from build123d import *

# Parameters (mm, degrees)
F0_W     = 152.4
F0_H     = 152.4
F0_R     = 3.175
F0_R_2   = 6.35
F1_DEPTH = 3.175
F2_R     = 5.08
F3_R     = 19.044803008
F3_R_2   = 6.35
F4_DEPTH = 0.7055555556


# Not quite as in the source:
# - a length typed as a fraction of an inch, garbled in the dataset ("3 / 203.2 mm" for 3/8 in), is restored


with BuildPart() as f1:
    # F0 (on Top) → F1 (new body)
    with BuildSketch(Plane.XY):
        with Locations((-1.8146978691, -1.1040684107)):
            Rectangle(F0_W, F0_H)
        with Locations((-67.6762834191, -67.5093614922)):
            Circle(F0_R, mode=Mode.SUBTRACT)
        with Locations((65.6737165809, -67.5093614922)):
            Circle(F0_R, mode=Mode.SUBTRACT)
        with Locations((-67.6762834191, 65.8406385078)):
            Circle(F0_R, mode=Mode.SUBTRACT)
        Circle(F0_R_2, mode=Mode.SUBTRACT)
        with Locations((65.6737165809, 65.8406385078)):
            Circle(F0_R, mode=Mode.SUBTRACT)
    extrude(amount=F1_DEPTH)

    # F2
    f2_edges = [f1.edges().sort_by_distance(p)[0] for p in [
        (74.385302, 75.095932, 1.5875),
        (-78.014698, 75.095932, 1.5875),
        (74.385302, -77.304068, 1.5875),
        (-78.014698, -77.304068, 1.5875),
    ]]
    fillet(f2_edges, radius=F2_R)

    # F3 (on face) → F4 (cut)
    with BuildSketch(Plane.XY.offset(3.175)):
        Circle(F3_R)
        Circle(F3_R_2, mode=Mode.SUBTRACT)
    extrude(amount=-F4_DEPTH, mode=Mode.SUBTRACT)


solid = f1.part
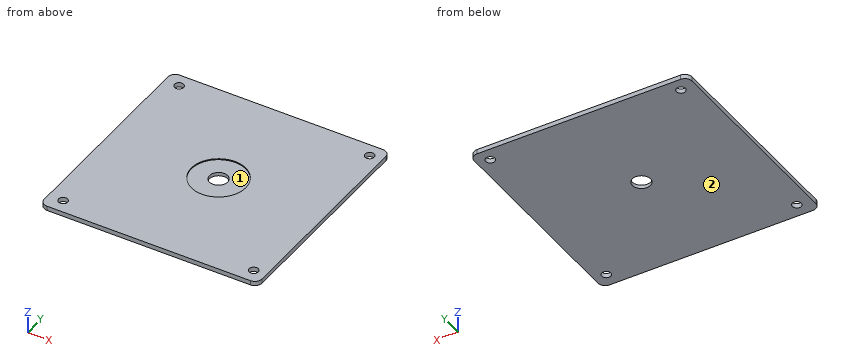
Can you work these out from the model? Positions are in its coordinate system, mm. Face numbers are marked on the shaded views. Round coordinates to 2 decimals unless told otherwise and drop trailing zeros. Write each loop counter-clockwise with the first axis right and the second up, starting at its lowest first coordinate (ties: lowest second). Pieces come first, ordered by that corner, then holes. Notation, with made-up numbers: M 42.25,-31 L 86.25,-31 A17 ccw 86.25,-10 Z; hole C 55,11.5 d6. An arc over 180 degrees is marked long. Use a Markdown table: item, result.
Item 1: For pin 1 Ø1.5 at (x, y) = (8, 11.5) entering from +Z, with a flat end and sliding along its axis, tell me the tip position at first contact or that it passes through.
Found:
| item | result |
|---|---|
| pin 1 | stops at z = 2.47 |
Item 2: If I drill on line 1 along Y through (x, z) = (-65.5, 2.65); line 2 along Y through (x, z) = (0, 1.55); line 3 along X through (y, z) = (8, 2.85), over which ranges is the centre line in solid material (lowest first)? Write a range as [from, to].
Found:
| item | result |
|---|---|
| line 1 | y = [-77.3, -69.82], [-65.2, 63.53], [68.15, 75.1] |
| line 2 | y = [-77.3, -6.35], [6.35, 75.1] |
| line 3 | x = [-78.01, -17.28], [17.28, 74.39] |
Item 3: I want a section at A-A (y = 0). List the corners of the cut face in (x, z) for me (3 decimals), and give its area (3 significant figures).
Found:
| item | result |
|---|---|
| outline | M -78.015,0 L -6.35,0 L -6.35,2.469 L -19.045,2.469 L -19.045,3.175 L -78.015,3.175 Z; M 6.35,0 L 74.385,0 L 74.385,3.175 L 19.045,3.175 L 19.045,2.469 L 6.35,2.469 Z |
| area | 426 mm2 |
Item 4: We'd pull the mould along X, two halves only. Please class the marked faces 1 and 2: released by +X, released by -X, zero draft, split by the parting line, or undercut.
Found:
| item | result |
|---|---|
| face 1 | undercut |
| face 2 | zero draft |
Item 5: I want a section at B-B (x = 0). List the corners of the cut face in (y, z) for me (3 decimals), and give its area (3 significant figures).
Found:
| item | result |
|---|---|
| outline | M -77.304,0 L -6.35,0 L -6.35,2.469 L -19.045,2.469 L -19.045,3.175 L -77.304,3.175 Z; M 6.35,0 L 75.096,0 L 75.096,3.175 L 19.045,3.175 L 19.045,2.469 L 6.35,2.469 Z |
| area | 426 mm2 |
